Here's how the part is built. I have some questions about the finished solid (model axes, mm). Give positions to 0.01 mm unless a question says otherwise; leave off trailing zeros. Order: outer loops, then holes, each group sorted by start corner. A loop starts at its lowest first (then second) coordinate and runs counter-clockwise, first axis right, second up.
from build123d import *

# Parameters (mm, degrees)
SKETCH1_R           = 0.89
SKETCH1_R_2         = 1.143
BOSS_EXTRUDE1_DEPTH = 1.5875


with BuildPart() as part:
    # Sketch1 → Boss-Extrude1 (new body)
    with BuildSketch(Plane(origin=(0, 0, 0), x_dir=(1, 0, 0), z_dir=(0, 1, 0))):
        with BuildLine():
            Line((-26.7, -6.35), (26.7, -6.35))
            Line((26.7, -6.35), (26.7, -1))
            ThreePointArc((26.7, -1), (25.7, 0), (26.7, 1))
            Line((26.7, 1), (26.7, 6.35))
            Line((26.7, 6.35), (-1.3, 6.35))
            add(Edge.make_bspline(
                [(-26.7, 2.65), (-1.3, 2.65), (-1.3, 6.35)],
                knots=[4.71238898, 4.71238898, 4.71238898, 6.283185307, 6.283185307, 6.283185307], degree=2, weights=[1, 0.707106781, 1]))
            Line((-26.7, 2.65), (-30.7, 2.65))
            Line((-30.7, 2.65), (-30.7, -6.35))
            Line((-30.7, -6.35), (-26.7, -6.35))
        make_face()
        with Locations(Location((-26.7, 0.51, 0), (0, 0, 270))):
            Circle(SKETCH1_R, mode=Mode.SUBTRACT)
        with Locations(Location((-26.7, -4.21, 0), (0, 0, 270))):
            Circle(SKETCH1_R, mode=Mode.SUBTRACT)
        with Locations(Location((2.7, 3.25, 0), (0, 0, 270))):
            Circle(SKETCH1_R_2, mode=Mode.SUBTRACT)
        with Locations(Location((2.7, -3.25, 0), (0, 0, 270))):
            Circle(SKETCH1_R_2, mode=Mode.SUBTRACT)
        with Locations(Location((22.7, 3.25, 0), (0, 0, 270))):
            Circle(SKETCH1_R_2, mode=Mode.SUBTRACT)
        with Locations(Location((22.7, -3.25, 0), (0, 0, 270))):
            Circle(SKETCH1_R_2, mode=Mode.SUBTRACT)
    extrude(amount=BOSS_EXTRUDE1_DEPTH)


solid = part.part
Q1. I need wall thicknesses on L1, parallel to X at y = 1.25, z = 3.25; L2, parallel to X at y = 0.55, z = 2.75; L3, parallel to X at y = 0.45, z = 4.25. Which ranges of each line are inside material? Lowest first, please.
Filled sheet:
L1: x = -30.7 to 1.56, 3.84 to 21.56, 23.84 to 26.7
L2: x = -30.7 to 1.67, 3.73 to 21.67, 23.73 to 26.7
L3: x = -30.7 to -27.59, -25.81 to 2.15, 3.25 to 22.15, 23.25 to 26.7
Q2. Thinking about a two-plate mould opening in Z: for faces 1 (the face through (-2, 1.588, 0)), 2 (the face through (-29, 1, -2.65)), 3 (the face through (-2, 1, 6.35)), 4 (the face through (25.7, 0.8, 0)), which applies, released by +Z, released by -Z, zero draft, split by the parting line, or undercut?
Filled sheet:
face 1: zero draft
face 2: released by -Z
face 3: released by +Z
face 4: undercut
Q3. If we section it at B-B on z = -0.51: List the corners of the cut face in (x, y) for me, plus the area to 3 significant figures.
Filled sheet:
outline: (-30.7, 0) - (-27.59, 0) - (-27.59, 1.59) - (-30.7, 1.59) - close; (-25.81, 0) - (25.84, 0) - (25.84, 1.59) - (-25.81, 1.59) - close
area: 86.9 mm2
Q4. I'm going to push a flat-ended pin straight in: P1, Ø3.5, axis at x = 22.7, z = -3.25, coming from the +Y side. Where does the tip first touch, or does it pass through?
Filled sheet:
P1: stops at y = 1.59
Q5. If we section it at C-C on y = 0.6: Give the number of separate pieces and of enclosed holes in the cut face, plus the area to 3 significant figures.
Filled sheet:
separate pieces: 1
enclosed holes: 6
area: 617 mm2
Q6. If we section it at A-A on x = 2.7: List the corners of the cut face in (y, z) for me, plus the area to 3 significant figures.
Filled sheet:
outline: (0, -6.35) - (1.59, -6.35) - (1.59, -4.39) - (0, -4.39) - close; (0, -2.11) - (1.59, -2.11) - (1.59, 2.11) - (0, 2.11) - close; (0, 4.39) - (1.59, 4.39) - (1.59, 6.35) - (0, 6.35) - close
area: 12.9 mm2
